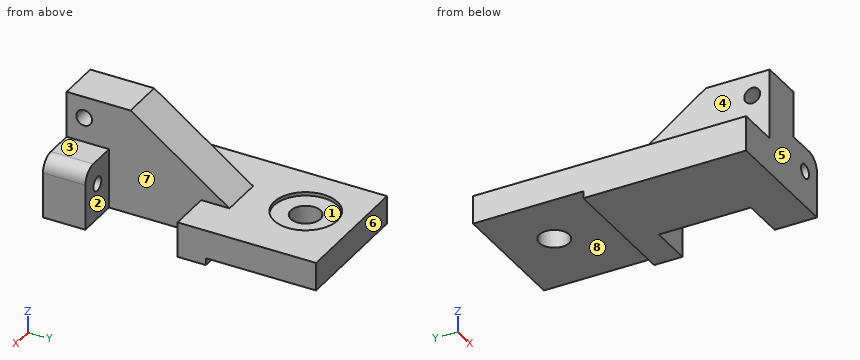
from build123d import *

# Parameters (mm, degrees)
F0_W            = 73.152
F0_H            = 15.875
F1_DEPTH        = 19.05
F3_D            = 7.112
F4_W            = 19.05
F4_H            = 26.924
F5_DEPTH        = 19.05
F7_D            = 6.35
F8_DEPTH        = 19.05
F9_DEPTH        = 49.53
F10_DEPTH       = 38.1
F11_DEPTH       = 12.7
F13_W           = 57.15
F13_H           = 49.53
F14_DEPTH       = 3.175
F16_D           = 13.335
F16_CBORE_D     = 28.575
F16_CBORE_DEPTH = 1.6002
F17_DEPTH       = 25.4


with BuildPart() as f1:
    # F0 (on Right) → F1 (new body)
    with BuildSketch(Plane.YZ):
        Polygon((0, 47.6504), (0, 15.875), (73.152, 15.875), (28.702, 47.6504), align=None)
        with Locations((36.576, 7.9375)):
            Rectangle(F0_W, F0_H)
    extrude(amount=F1_DEPTH)

    # F3 (through all)
    with Locations(Plane.YZ.offset(19.05)):
        with Locations((7.874, 37.9984)):
            Hole(F3_D / 2)

    # F4 (on face) → F5 (join)
    with BuildSketch(Plane.YZ.offset(19.05)):
        with Locations((9.525, 13.462)):
            Rectangle(F4_W, F4_H)
    extrude(amount=F5_DEPTH)

    # F7 (through all)
    with Locations(Plane(origin=(0, 19.05, 0), x_dir=(-1, 0, 0), z_dir=(0, 1, 0))):
        with Locations((-28.448, 16.002)):
            Hole(F7_D / 2)


with BuildPart() as f8:
    # F0 (on Right) → F8 (new body)
    with BuildSketch(Plane.YZ):
        with Locations((36.576, 7.9375)):
            Rectangle(F0_W, F0_H)
    extrude(amount=-F8_DEPTH)


with BuildPart() as f9:
    # F9 (new): a face of the model
    f9_faces = [f8.part.faces().sort_by_distance(p)[0] for p in [
        (-9.525, 73.152, 7.9375),
    ]]
    extrude(f9_faces, amount=F9_DEPTH)


with BuildPart() as f10:
    # F10 (new): a face of the model
    f10_faces = [f9.part.faces().sort_by_distance(p)[0] for p in [
        (0, 97.917, 7.9375),
    ]]
    extrude(f10_faces, amount=F10_DEPTH)


with BuildPart() as f11:
    # F11 (new): a face of the model
    f11_faces = [f10.part.faces().sort_by_distance(p)[0] for p in [
        (19.05, 73.152, 7.9375),
    ]]
    extrude(f11_faces, amount=F11_DEPTH)


with BuildPart() as f1_1:
    add(f1.part)

    # F12: union F8, F9, F10, F11
    add(f8.part)
    add(f9.part)
    add(f10.part)
    add(f11.part)

    # F13 (on Top) → F14 (cut)
    with BuildSketch(Plane.XY):
        with Locations((9.525, 97.917)):
            Rectangle(F13_W, F13_H)
    extrude(amount=F14_DEPTH, mode=Mode.SUBTRACT)

    # F16 (through all)
    with Locations(Plane.XY.offset(15.875)):
        with Locations((6.35, 100.33)):
            CounterBoreHole(F16_D / 2, F16_CBORE_D / 2, F16_CBORE_DEPTH)

    # F6 (on face) → F17 (cut)
    with BuildSketch(Plane(origin=(0, 19.05, 0), x_dir=(-1, 0, 0), z_dir=(0, 1, 0))):
        with BuildLine():
            ThreePointArc((-38.1, 20.574), (-36.2401280605, 25.0641280605), (-31.75, 26.924))
            Line((-31.75, 26.924), (-38.1, 26.924))
            Line((-38.1, 26.924), (-38.1, 20.574))
        make_face()
    extrude(amount=-F17_DEPTH, mode=Mode.SUBTRACT)


solid = f1_1.part
For this review, take the finished solid that the model builds, in its own axes (mm). Face numbers are marked on the shaded views. A direction names the side the tool comes from. Round coordinates to 2 decimals unless told otherwise and drop trailing zeros. Order: outer loops, then holes, each group sorted by start corner. A loop starts at its lowest first (then second) coordinate and runs counter-clockwise, first axis right, second up. Notation, with made-up numbers: M 50,69 L 90,69 A20 ccw 90,79 Z; hole C 55.5,69.5 d3. An arc over 180 degrees is marked long. Write each question's results on one line, items separated by ' | '. Start each with the question number.
1. Clearance check with flat-ended pins moving along their axes: pin 1 Ø1 at (x, z) = (12.5, 40.5) entering from -Y; pin 2 Ø21.5 at (x, y) = (6.35, 100.33) entering from +Z; pin 3 Ø6.5 at (x, y) = (24, 6.5) entering from +Z; pin 4 Ø8 at (y, z) = (7.87, 38) entering from +X. State where each tip first meets the part, or that it passes through.
2. Tool access review of the marked faces 1, 2, 3 and 4: name each direction out of +Z, -Z, +X, -X, +Y, -Y from which nothing blocks a thin tool from reaching the whole face with its end or side.
3. Add section A-A (x = 6.35). State the section outline as (y, z) points (1 decimal).
4. Draft analysis for pull direction Y (two halves, no side actions). For the marked faces 5, 6, 7 and 8, state which applies: pulls with the +Y half, pulls with the -Y half, needs draft (parallel to the pull), parting line crosses it, or undercut.
5. Add section D-D (x = -14). State the section outline as (y, z) points (3 decimals).
6. Add section C-C (z = 36.5). State the section outline as (x, y) points, then the cut area to 3 significant figures.
7. To check wall thickness, follow L1, parallel to Z at x = -15, y = 110 (3 decimals); L2, parallel to X at y = 14, z = 44; L3, parallel to Y at x = 28, z = 3. State the ranges of each line that lie inside material, in increasing order. Write a range as [from, to].
Output values:
1) pin 1: y = 0 | pin 2: z = 14.27 | pin 3: z = 26.92 | pin 4: x = 19.05
2) face 1: +Z | face 2: +Z, -Z, +X | face 3: +Z, +X, +Y, -Y | face 4: +Z, -X, +Y, -Y
3) outline: M 0,0 L 73.2,0 L 73.2,3.2 L 93.7,3.2 L 93.7,14.3 L 86,14.3 L 86,15.9 L 73.2,15.9 L 28.7,47.7 L 0,47.7 Z; M 107,3.2 L 122.7,3.2 L 122.7,15.9 L 114.6,15.9 L 114.6,14.3 L 107,14.3 Z; hole C 7.9,38 d7.1
4) face 5: pulls with the -Y half | face 6: pulls with the +Y half | face 7: undercut | face 8: needs draft
5) outline: M 0,0 L 73.152,0 L 73.152,3.175 L 122.682,3.175 L 122.682,15.875 L 0,15.875 Z
6) outline: M 0,0 L 19.05,0 L 19.05,4.65 L 0,4.65 Z; M 0,11.1 L 19.05,11.1 L 19.05,44.3 L 0,44.3 Z | area: 721 mm^2
7) L1: [3.175, 15.875] | L2: [0, 19.05] | L3: [0, 19.05], [60.45, 73.15]
